Check sheet for the modelled part. Datum: model origin and axes. Units: mm. A direction names the side the tool comes from. Round coordinates to 2 decimals unless told otherwise and drop trailing zeros. Write each loop counter-clockwise with the first axis right and the second up, starting at its lowest first coordinate (ties: lowest second). Pieces come first, ordered by that corner, then holes. Notation, with made-up numbers: M 70,2 L 82,2 A7 cw 82,15 Z; hole C 83,-39.5 d11. An arc over 180 degrees is marked long. One line per item, written item: value.
from build123d import *

# Parameters (mm, degrees)
SKETCH_1_W          = 25
SKETCH_1_H          = 90
EXTRUDE_1_DEPTH     = 3
SKETCH_3_R          = 1.75
CUT_EXTRUDE_1_DEPTH = 4
CUT_EXTRUDE_2_DEPTH = 4


with BuildPart() as part:
    # 草图1 → 凸台-拉伸1 (new body)
    with BuildSketch(Plane.XY):
        Rectangle(SKETCH_1_W, SKETCH_1_H)
    extrude(amount=EXTRUDE_1_DEPTH)

    # 草图3 → 切除-拉伸1 (cut, through all)
    with BuildSketch(Plane.XY.offset(3)):
        with Locations((0, 38)):
            Circle(SKETCH_3_R)
        with Locations((0, 24)):
            Circle(SKETCH_3_R)
        with Locations((-5, -35)):
            Circle(SKETCH_3_R)
        with Locations((5, -35)):
            Circle(SKETCH_3_R)
    extrude(amount=-CUT_EXTRUDE_1_DEPTH, mode=Mode.SUBTRACT)

    # 草图4 → 切除-拉伸2 (cut, through all)
    with BuildSketch(Plane.XY.offset(3)):
        with BuildLine():
            Line((-5, 2.5), (5, 2.5))
            ThreePointArc((5, 2.5), (7.5, 0), (5, -2.5))
            Line((5, -2.5), (-5, -2.5))
            ThreePointArc((-5, -2.5), (-7.5, 0), (-5, 2.5))
        make_face()
    extrude(amount=-CUT_EXTRUDE_2_DEPTH, mode=Mode.SUBTRACT)


solid = part.part
Q1. Sectioned sample at C-C on x = 0. Enter the section's corners in (y, z).
Completed:
outline: M -45,0 L -2.5,0 L -2.5,3 L -45,3 Z; M 2.5,0 L 22.25,0 L 22.25,3 L 2.5,3 Z; M 25.75,0 L 36.25,0 L 36.25,3 L 25.75,3 Z; M 39.75,0 L 45,0 L 45,3 L 39.75,3 Z
Q2. Sectioned sample at B-B on y = -35. Enter the section's corners in (x, z).
Completed:
outline: M -12.5,0 L -6.75,0 L -6.75,3 L -12.5,3 Z; M -3.25,0 L 3.25,0 L 3.25,3 L -3.25,3 Z; M 6.75,0 L 12.5,0 L 12.5,3 L 6.75,3 Z
Q3. Draft check along X on faces 1 (the cylindrical face through (-6.75, -34.92, 1.52)), 2 (the flat face through (-9, 1, 3)), 3 (the flat face through (-12.5, -1, 1)). Enter one of: pulls with the +X half, pulls with the -X half, needs draft (parallel to the pull), parting line crosses it, or undercut.
Completed:
face 1: undercut
face 2: needs draft
face 3: pulls with the -X half
Q4. Scan lines: line 1 (Y direction, x = 0, z = 0.95); line 2 (Y direction, x = -5, z = 2.1); line 3 (Y direction, x = -4, z = 0.3). Record each from-to range of solid material in increasing order. Write a range as [from, to].
Completed:
line 1: [-45, -2.5], [2.5, 22.25], [25.75, 36.25], [39.75, 45]
line 2: [-45, -36.75], [-33.25, -2.5], [2.5, 45]
line 3: [-45, -36.44], [-33.56, -2.5], [2.5, 45]
Q5. Sectioned sample at D-D on z = 0.55. Enter the section's corners in (x, y).
Completed:
outline: M -12.5,-45 L 12.5,-45 L 12.5,45 L -12.5,45 Z; hole C -5,-35 d3.5; hole M -5,-2.5 L 5,-2.5 A2.5 ccw 5,2.5 L -5,2.5 A2.5 ccw Z; hole C 0,24 d3.5; hole C 0,38 d3.5; hole C 5,-35 d3.5
Q6. Sectioned sample at A-A on y = 38. Enter the section's corners in (x, z).
Completed:
outline: M -12.5,0 L -1.75,0 L -1.75,3 L -12.5,3 Z; M 1.75,0 L 12.5,0 L 12.5,3 L 1.75,3 Z
Q7. Access from +Z, -Z, +X, -X, +Y, -Y to the whole of each face (thin tool, end or side, straight path). Record for faces 4 (the flat face through (-9, 1, 0)), 5 (the cylindrical face through (-7.5, -0.1, 1.5)).
Completed:
face 4: -Z, +X, -X, +Y, -Y
face 5: +Z, -Z
Q8. Depth check by flat-ended pin: P1, Ø4.5, axis at x = 0, y = 38, coming from the +Z side. Enter the tip coordinate at first touch or a pass-through.
Completed:
P1: z = 3
